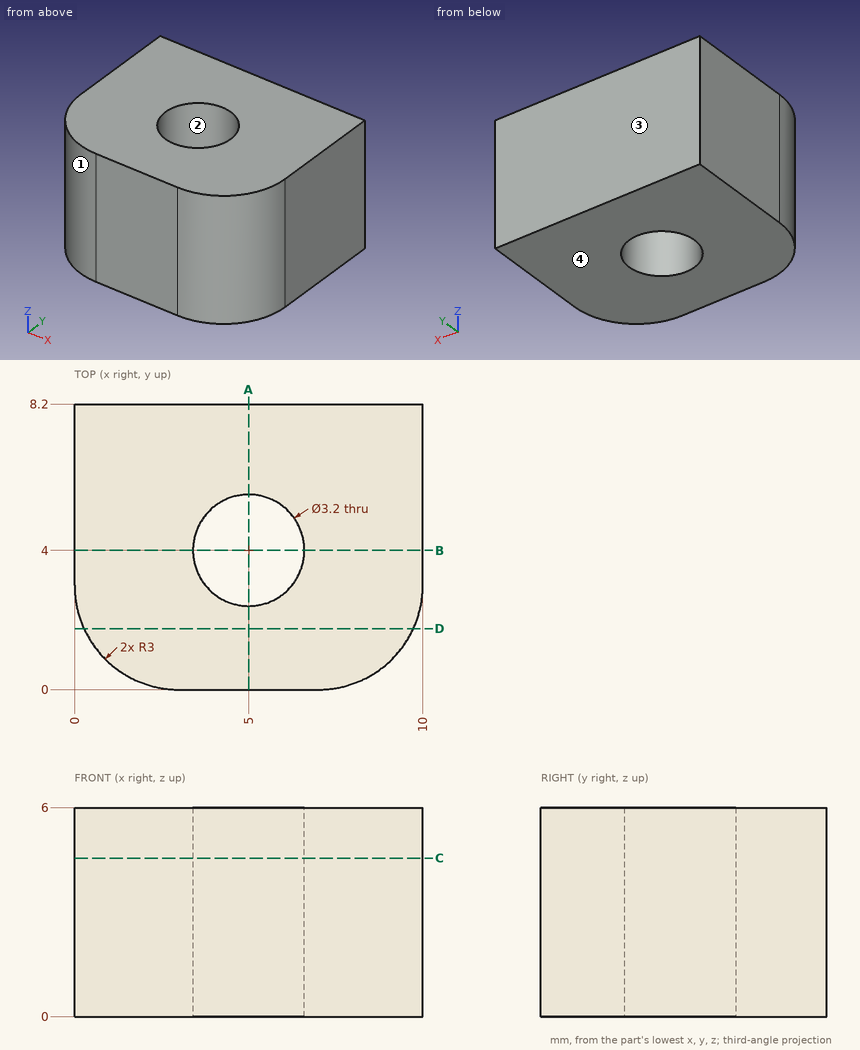
Design review of the part shown in the three views and the two pictorial views. Dimensions are in mm from the part's minimum x, y and z. Coordinates: 2 decimals unless noted, no trailing zeros. Loops run counter-clockwise (first coordinate to the right, second up) from the corner with the lowest first, then second, coordinate; pieces in that order, holes last.
Q1. We need section D-D on y = 1.75. State the section outline as (x, z) points, and give its area (3 significant figures).
Reported:
outline: (0.27, 0) - (9.73, 0) - (9.73, 6) - (0.27, 6) - close
area: 56.7 mm2
Q2. We need section C-C on z = 4.55. State the section outline as (x, y) points.
Reported:
outline: (0, 3) arc R3 ccw to (3, 0) - (7, 0) arc R3 ccw to (10, 3) - (10, 8.2) - (0, 8.2) - close; hole circle Ø3.2 at (5, 4)
Q3. We need section B-B on y = 4. State the section outline as (x, z) points, and give its area (3 significant figures).
Reported:
outline: (0, 0) - (3.4, 0) - (3.4, 6) - (0, 6) - close; (6.6, 0) - (10, 0) - (10, 6) - (6.6, 6) - close
area: 40.8 mm2
Q4. The part is to be moulded in two halves that separate along Y. For the marked faces 1, 2, 3 and 4, say which applies: +Y half, -Y half, draft (parallel to the pull), parting line (faces both ways), or undercut.
Reported:
face 1: -Y half
face 2: undercut
face 3: +Y half
face 4: draft
Q5. We need section A-A on x = 5. State the section outline as (y, z) points.
Reported:
outline: (0, 0) - (2.4, 0) - (2.4, 6) - (0, 6) - close; (5.6, 0) - (8.2, 0) - (8.2, 6) - (5.6, 6) - close
Q6. To check wall thickness, follow line 1 (Y direction, x = 5, z = 3.1); line 2 (Y direction, x = 5.5, z = 2.25); line 3 (Y direction, x = 2.25, z = 4.3). State the ranges of each line that lie inside material, in increasing order.
Reported:
line 1: y = 0 to 2.4, 5.6 to 8.2
line 2: y = 0 to 2.48, 5.52 to 8.2
line 3: y = 0.1 to 8.2
